The listing builds one solid part. Answer for the finished solid, in the listing's coordinates (mm). A direction names the side the tool comes from. Give positions to 0.01 mm unless a question says otherwise; leave off trailing zeros. Write each loop counter-clockwise with the first axis right and the second up, starting at its lowest first coordinate (ties: lowest second). Pieces come first, ordered by that corner, then holes. Notation, with made-up numbers: M 73,35 L 86,35 A25 cw 86,65 Z; hole C 79.25,-30 d8. An arc over 180 degrees is marked long. Answer as a JSON object with one key per item and string values.
```python
from build123d import *

# Parameters (mm, degrees)
F0_W     = 8
F0_H     = 2
F1_DEPTH = 2
F2_DEPTH = 1.3
F3_START = -1.3
F3_DEPTH = 2


with BuildPart() as f1:
    # F0 (on Top) → F1 (new body)
    with BuildSketch(Plane.XY):
        with BuildLine():
            ThreePointArc((-2.5, 19.66), (0, 22.16), (2.5, 19.66))
            Line((2.5, 19.66), (4, 19.66))
            Line((4, 19.66), (4, 19.422723854))
            ThreePointArc((4, 19.422723854), (4.4045880471, 20.3405322852), (4.8541019662, 21.2371933364))
            Line((4.8541019662, 21.2371933364), (0, 24.7639048501))
            Line((0, 24.7639048501), (-4.8541019662, 21.2371933364))
            ThreePointArc((-4.8541019662, 21.2371933364), (-4.4045880471, 20.3405322852), (-4, 19.422723854))
            Line((-4, 19.422723854), (-4, 19.66))
            Line((-4, 19.66), (-2.5, 19.66))
        make_face()
        with BuildLine():
            ThreePointArc((2.5, 12.7140819367), (1.8321382954, 15.2643852238), (0, 17.16))
            ThreePointArc((0, 17.16), (-1.8321382954, 15.2643852238), (-2.5, 12.7140819367))
            ThreePointArc((-2.5, 12.7140819367), (-2.7688401868, 8.2742164407), (-4, 4))
            Line((-4, 4), (-4, 2))
            Line((-4, 2), (4, 2))
            Line((4, 2), (4, 4))
            ThreePointArc((4, 4), (2.7688401868, 8.2742164407), (2.5, 12.7140819367))
        make_face()
        with Locations((0, 1)):
            Rectangle(F0_W, F0_H)
        with BuildLine():
            ThreePointArc((0, 17.16), (-1.767766953, 17.892233047), (-2.5, 19.66))
            Line((-2.5, 19.66), (-2.5, 12.7140819367))
            ThreePointArc((-2.5, 12.7140819367), (-1.8321382954, 15.2643852238), (0, 17.16))
        make_face()
        with BuildLine():
            Line((2.5, 12.7140819367), (2.5, 19.66))
            ThreePointArc((2.5, 19.66), (1.767766953, 17.892233047), (0, 17.16))
            ThreePointArc((0, 17.16), (1.8321382954, 15.2643852238), (2.5, 12.7140819367))
        make_face()
        with BuildLine():
            Line((-2.5, 12.7140819367), (-2.5, 19.66))
            Line((-2.5, 19.66), (-4, 19.66))
            Line((-4, 19.66), (-4, 19.422723854))
            ThreePointArc((-4, 19.422723854), (-2.9634091525, 16.1324823732), (-2.5, 12.7140819367))
        make_face()
        with BuildLine():
            Line((4, 19.66), (2.5, 19.66))
            Line((2.5, 19.66), (2.5, 12.7140819367))
            ThreePointArc((2.5, 12.7140819367), (2.9634091525, 16.1324823732), (4, 19.422723854))
            Line((4, 19.422723854), (4, 19.66))
        make_face()
    extrude(amount=F1_DEPTH)

    # F0 (on Top) → F2 (join)
    with BuildSketch(Plane.XY):
        with Locations((0, 1)):
            Rectangle(F0_W, F0_H)
    extrude(amount=-F2_DEPTH)

    # F0 (on Top) → F3 (join)
    with BuildSketch(Plane.XY.offset(F3_START)):
        with BuildLine():
            ThreePointArc((2.5, 12.7140819367), (1.8321382954, 15.2643852238), (0, 17.16))
            ThreePointArc((0, 17.16), (-1.8321382954, 15.2643852238), (-2.5, 12.7140819367))
            ThreePointArc((-2.5, 12.7140819367), (-2.7688401868, 8.2742164407), (-4, 4))
            Line((-4, 4), (-4, 2))
            Line((-4, 2), (4, 2))
            Line((4, 2), (4, 4))
            ThreePointArc((4, 4), (2.7688401868, 8.2742164407), (2.5, 12.7140819367))
        make_face()
        with Locations((0, 1)):
            Rectangle(F0_W, F0_H)
    extrude(amount=-F3_DEPTH)


solid = f1.part
```
1. A cutting plane is placed at B-B, the plane x = -3.25. Give the vertices of the cut face in (y, z).
Verdict:
{"outline": "M 0,-3.3 L 6.16,-3.3 L 6.16,-1.3 L 2,-1.3 L 2,0 L 6.16,0 L 6.16,2 L 0,2 Z; M 17.26,0 L 22.4,0 L 22.4,2 L 17.26,2 Z"}
2. Flat-ended cylindrical pins translate along their axes: pin 1 (2 mm diameter, centred on y = 1, z = -2, fed in from +X); pin 2 (2 mm diameter, centred on y = 11.5, z = -1, fed in from +X); pin 3 (1.5 mm diameter, centred on y = 13, z = 1.5, fed in from -X); pin 4 (5 mm diameter, centred on x = 0.5, y = 17.5, fed in from -Z). Find the tip coordinate at first contact, or state that the pin passes through.
Verdict:
{"pin 1": "stops at x = 4", "pin 2": "stops at x = 2.51", "pin 3": "stops at x = -2.58", "pin 4": "stops at z = -3.3"}
3. A cutting plane is placed at D-D, the plane z = -2.2. Give the vertices of the cut face in (x, y).
Verdict:
{"outline": "M -4,0 L 4,0 L 4,4 A20.26 cw 2.5,12.71 A5.2 ccw 0,17.16 A5.2 ccw -2.5,12.71 A20.26 cw -4,4 Z"}
4. For faces 1 (the flat face through (0, 11, 0)), 2 (the cylindrical face through (1.85, 15.23, -2.29)), 3 (the flat face through (-4, 1.6, -0.6)), 4 (the flat face through (4, 1.5, -0.6)), determine the directions among +Z, -Z, +X, -X, +Y, -Y from which every point of the face is accessible in a straight line to the end or side of a thin tool.
Verdict:
{"face 1": "+X, -X, +Y", "face 2": "-Z, +X, +Y", "face 3": "+Z, -Z, -X, -Y", "face 4": "+Z, -Z, +X, -Y"}
5. Consider line 1 along Z through (x, y) = (1, 14.25); line 2 along Y through (x, z) = (-1, -0.75); line 3 along Y through (x, z) = (-0.5, 0.65). Determine where each line is inside the solid, lowest interval first.
Verdict:
{"line 1": "z = -3.3 to -1.3, 0 to 2", "line 2": "y = 0 to 2", "line 3": "y = 0 to 17.21, 22.11 to 24.4"}
6. A cutting plane is placed at A-A, the plane y = 2.5. Give the vertices of the cut face in (x, z).
Verdict:
{"outline": "M -4,-3.3 L 4,-3.3 L 4,-1.3 L -4,-1.3 Z; M -4,0 L 4,0 L 4,2 L -4,2 Z"}
7. A cutting plane is placed at C-C, the plane z = 0.3. Give the vertices of the cut face in (x, y).
Verdict:
{"outline": "M -4.85,21.24 A20.26 cw -4,4 L -4,0 L 4,0 L 4,4 A20.26 cw 4.85,21.24 L 0,24.76 Z; hole C 0,19.66 d5"}
8. The mould has two halves that part along Y. Classify faces 5 (the flat face through (0, 0, -1)), 6 (the cylindrical face through (-2.758, 8.336, -2.286)), 7 (the flat face through (0, 8, -1.3)), 8 (the cylindrical face through (2.78, 8.21, -2.29)): released by +Y, released by -Y, zero draft, split by the parting line, or undercut.
Verdict:
{"face 5": "released by -Y", "face 6": "undercut", "face 7": "zero draft", "face 8": "undercut"}
